Read the model definition and answer for the solid it produces. Units are mm, in the model's axes. Face numbers are marked on the shaded views. A direction names the side the tool comes from. Give positions to 0.01 mm unless a question says otherwise; leave off trailing zeros. Write each loop counter-clockwise with the first axis right and the second up, starting at its lowest first coordinate (ties: lowest second). Pieces come first, ordered by that corner, then holes. Notation, with made-up numbers: M 86,50.5 L 131,50.5 A30 cw 131,79.5 Z; hole C -24.75,-21 d11. An arc over 180 degrees is marked long. Write each question's results on one line, items separated by ' | '. Start each with the question number.
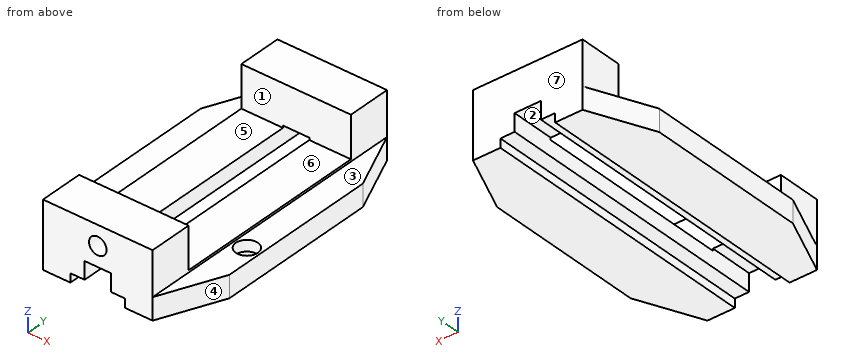
```python
from build123d import *

# Parameters (mm, degrees)
F1_DEPTH  = 30
F2_W      = 12
F2_H      = 130
F3_DEPTH  = 20
F4_W      = 50
F4_H      = 90
F5_DEPTH  = 19
F7_DEPTH  = 130.001
F8_R      = 4
F9_DEPTH  = 20
F10_R     = 5
F11_DEPTH = 5


with BuildPart() as f1:
    # F0 (on Top) → F1 (new body)
    with BuildSketch(Plane.XY):
        Polygon((37, 37), (25, 65), (-25, 65), (-37, 37), (-37, -37), (-25, -65), (25, -65), (37, -37), align=None)
    extrude(amount=F1_DEPTH)

    # F2 (on face) → F3 (cut)
    with BuildSketch(Plane.XY.offset(30)):
        with Locations((31, 0)):
            Rectangle(F2_W, F2_H)
        with Locations((-31, 0)):
            Rectangle(F2_W, F2_H)
    extrude(amount=-F3_DEPTH, mode=Mode.SUBTRACT)

    # F4 (on face) → F5 (cut)
    with BuildSketch(Plane.XY.offset(30)):
        Rectangle(F4_W, F4_H)
    extrude(amount=-F5_DEPTH, mode=Mode.SUBTRACT)

    # F6 (on face) → F7 (cut, through all)
    with BuildSketch(Plane.XZ.offset(65)):
        Polygon((-12.5, 4), (-12.5, 0), (12.5, 0), (12.5, 4), (6, 4), (6, 12), (-6, 12), (-6, 4), align=None)
    extrude(amount=-F7_DEPTH, mode=Mode.SUBTRACT)

    # F8 (on face) → F9 (cut, through all)
    with BuildSketch(Plane.XZ.offset(65)):
        with Locations((0, 21)):
            Circle(F8_R)
    extrude(amount=-F9_DEPTH, mode=Mode.SUBTRACT)

    # F10 (on face) → F11 (cut)
    with BuildSketch(Plane.XY.offset(10)):
        with Locations((31, -20)):
            Circle(F10_R)
    extrude(amount=-F11_DEPTH, mode=Mode.SUBTRACT)


solid = f1.part
```
Item 1: Section D-D, the plane z = 15.75 is taken. Determine the outline of the cut face in (x, y), then the cut area to 3 significant figures.
Item 2: Section C-C, the plane x = 0 is taken. Determine the outline of the cut face in (y, z), then the cut area to 3 significant figures.
Item 3: Section B-B, the plane z = 7.75 is taken. Determine the outline of the cut face in (x, y).
Item 4: Given P1, Ø1.5, axis at x = -7, y = 16.5, coming from the +Z side; P2, Ø6, axis at x = -0.5, y = -59, coming from the -Z side; P3, Ø2, axis at x = 8, y = 0.5, coming from the -Z side; P4, Ø4, axis at x = -27.5, z = 20.5, coming from the -Y side, each flat-ended and moving along its own axis, determine where each tip first touches the part or whether it passes through.
Item 5: Straight lines are drawn through the part: line 1 (Y direction, x = 9.5, z = 18.5); line 2 (X direction, y = 28.5, z = 2.5); line 3 (X direction, y = 30.5, z = 9.25). For each, find the intervals that lie inside material, in ascending order.
Item 6: Section A-A, the plane y = 10.5 is taken. Determine the outline of the cut face in (x, z).
Item 7: For the marked faces 1, 2 and 3, determine the directions among +Z, -Z, +X, -X, +Y, -Y from which every point of the face is accessible in a straight line to the end or side of a thin tool.
Item 8: Determine the mould class of the marked faces 4, 5, 6 and 7 for opening direction Y: +Y half, -Y half, draft (parallel to the pull), parting line (faces both ways), or undercut.
Worked out:
1) outline: M -25,-65 L 25,-65 L 25,-45 L -25,-45 Z; M -25,45 L 25,45 L 25,65 L -25,65 Z | area: 2,000 mm²
2) outline: M -65,12 L -45,12 L -45,17 L -65,17 Z; M -65,25 L -45,25 L -45,30 L -65,30 Z; M 45,12 L 65,12 L 65,30 L 45,30 Z | area: 560 mm²
3) outline: M -37,-37 L -25,-65 L -6,-65 L -6,65 L -25,65 L -37,37 Z; M 6,-65 L 25,-65 L 37,-37 L 37,37 L 25,65 L 6,65 Z; hole C 31,-20 d10
4) P1: stops at z = 11 | P2: stops at z = 12 | P3: stops at z = 4 | P4: passes through
5) line 1: y = -65 to -45, 45 to 65 | line 2: x = -37 to -12.5, 12.5 to 37 | line 3: x = -37 to -6, 6 to 37
6) outline: M -37,0 L -12.5,0 L -12.5,4 L -6,4 L -6,11 L -25,11 L -25,10 L -37,10 Z; M 6,4 L 12.5,4 L 12.5,0 L 37,0 L 37,10 L 25,10 L 25,11 L 6,11 Z
7) face 1: +Z, +X, -X | face 2: -Z, +Y, -Y | face 3: +Z, +X, +Y, -Y
8) face 4: -Y half | face 5: undercut | face 6: undercut | face 7: +Y half
